from build123d import *

# Parameters (mm, degrees)
BOSS_EXTRUDE1_DEPTH = 1.5875
CUT_EXTRUDE1_DEPTH  = 5.08


with BuildPart() as part:
    # Sketch2 → Boss-Extrude1 (new body, symmetric)
    with BuildSketch(Plane.XY):
        Polygon((-31.75, -76.2), (-95.25, -76.2), (-31.75, 76.2), (31.75, 76.2), (31.75, -76.2), align=None)
    extrude(amount=BOSS_EXTRUDE1_DEPTH, both=True)

    # Sketch3 → Cut-Extrude1 (cut)
    with BuildSketch(Plane.XY.offset(1.5875)):
        with BuildLine():
            Line((-60.897552188, -22.755874748), (-42.901529882, -65.946328282))
            ThreePointArc((-42.901529882, -65.946328282), (-43.158162937, -68.594558042), (-45.503977694, -69.85))
            Line((-45.503977694, -69.85), (-81.496022306, -69.85))
            ThreePointArc((-81.496022306, -69.85), (-83.841837063, -68.594558042), (-84.098470118, -65.946328282))
            Line((-84.098470118, -65.946328282), (-66.102447812, -22.755874748))
            ThreePointArc((-66.102447812, -22.755874748), (-63.5, -21.020909541), (-60.897552188, -22.755874748))
        make_face()
        with BuildLine():
            ThreePointArc((-25.4, 30.353407686), (-23.133595378, 33.117976889), (-19.978233725, 31.437760941))
            Line((-19.978233725, 31.437760941), (-7.330980523, 1.084353255))
            ThreePointArc((-7.330980523, 1.084353255), (-7.114109872, 0), (-7.330980523, -1.084353255))
            Line((-7.330980523, -1.084353255), (-19.978233725, -31.437760941))
            ThreePointArc((-19.978233725, -31.437760941), (-23.133595378, -33.117976889), (-25.4, -30.353407686))
            Line((-25.4, -30.353407686), (-25.4, 30.353407686))
        make_face()
        with BuildLine():
            ThreePointArc((-20.598470118, 65.946328282), (-20.341837063, 68.594558042), (-17.996022306, 69.85))
            Line((-17.996022306, 69.85), (17.996022306, 69.85))
            ThreePointArc((17.996022306, 69.85), (20.341837063, 68.594558042), (20.598470118, 65.946328282))
            Line((20.598470118, 65.946328282), (2.602447812, 22.755874748))
            ThreePointArc((2.602447812, 22.755874748), (0, 21.020909541), (-2.602447812, 22.755874748))
            Line((-2.602447812, 22.755874748), (-20.598470118, 65.946328282))
        make_face()
        with BuildLine():
            ThreePointArc((-2.602447812, -22.755874748), (0, -21.020909541), (2.602447812, -22.755874748))
            Line((2.602447812, -22.755874748), (20.598470118, -65.946328282))
            ThreePointArc((20.598470118, -65.946328282), (20.341837063, -68.594558042), (17.996022306, -69.85))
            Line((17.996022306, -69.85), (-17.996022306, -69.85))
            ThreePointArc((-17.996022306, -69.85), (-20.341837063, -68.594558042), (-20.598470118, -65.946328282))
            Line((-20.598470118, -65.946328282), (-2.602447812, -22.755874748))
        make_face()
        with BuildLine():
            Line((-38.1, 30.353407686), (-38.1, -30.353407686))
            ThreePointArc((-38.1, -30.353407686), (-40.366404622, -33.117976889), (-43.521766275, -31.437760941))
            Line((-43.521766275, -31.437760941), (-56.169019477, -1.084353255))
            ThreePointArc((-56.169019477, -1.084353255), (-56.385890128, 0), (-56.169019477, 1.084353255))
            Line((-56.169019477, 1.084353255), (-43.521766275, 31.437760941))
            ThreePointArc((-43.521766275, 31.437760941), (-40.366404622, 33.117976889), (-38.1, 30.353407686))
        make_face()
        with BuildLine():
            Line((25.4, -30.353407686), (25.4, 30.353407686))
            ThreePointArc((25.4, 30.353407686), (23.133595378, 33.117976889), (19.978233725, 31.437760941))
            Line((19.978233725, 31.437760941), (7.330980523, 1.084353255))
            ThreePointArc((7.330980523, 1.084353255), (7.114109872, 0), (7.330980523, -1.084353255))
            Line((7.330980523, -1.084353255), (19.978233725, -31.437760941))
            ThreePointArc((19.978233725, -31.437760941), (23.133595378, -33.117976889), (25.4, -30.353407686))
        make_face()
    extrude(amount=-CUT_EXTRUDE1_DEPTH, mode=Mode.SUBTRACT)


solid = part.part
Design review of the part built by this model. Coordinates are the model's own, in mm. Coordinates: 2 decimals unless noted, no trailing zeros. Order: outer loops, then holes, each group sorted by start corner. A loop starts at its lowest first (then second) coordinate and runs counter-clockwise, first axis right, second up.
Item 1: Take a section at B-B, the plane x = 0.5. Write out the cut boundary in (y, z).
Item 2: Take a section at A-A, the plane y = -46. Write out the cut boundary in (x, z).
Item 3: Take a section at C-C, the plane z = -0.25. Count the separate pieces of the cut face and the enclosed holes in it, then the cut area to 3 significant figures.
Item 4: For pin 1 Ø1.6 at (x, z) = (-63.5, -0.5) entering from +Y; pin 2 Ø1.6 at (y, z) = (-14, 0.5) entering from -X, all flat-tipped, find the tip position at first contact; note any pin that passes through.
Item 5: The part is to be moulded in two halves that separate along X. For faces 1 (the flat face through (-52.026, -44.049, 0.022)), 2 (the flat face through (-63.944, -1.067, 0.022)), say which applies: pulls with the +X half, pulls with the -X half, needs draft (parallel to the pull), parting line crosses it, or undercut.
Item 6: For line 1 (X direction, y = -7.5, z = -1.15) (3 decimals); line 2 (X direction, y = 4, z = 1.1); line 3 (X direction, y = -67, z = 1), list the stretches that pass through material, from the lowest coordinate up.
Item 7: Take a section at D-D, the plane y = -28. Write out the cut boundary in (x, z).
The answers:
1. outline: (-76.2, -1.59) - (-69.85, -1.59) - (-69.85, 1.59) - (-76.2, 1.59) - close; (-21.07, -1.59) - (21.07, -1.59) - (21.07, 1.59) - (-21.07, 1.59) - close; (69.85, -1.59) - (76.2, -1.59) - (76.2, 1.59) - (69.85, 1.59) - close
2. outline: (-82.67, -1.59) - (-75.79, -1.59) - (-75.79, 1.59) - (-82.67, 1.59) - close; (-51.21, -1.59) - (-12.29, -1.59) - (-12.29, 1.59) - (-51.21, 1.59) - close; (12.29, -1.59) - (31.75, -1.59) - (31.75, 1.59) - (12.29, 1.59) - close
3. separate pieces: 1
3. enclosed holes: 6
3. area: 8,720 mm2
4. pin 1: stops at y = 1.92
4. pin 2: stops at x = -69.67
5. face 1: undercut
5. face 2: pulls with the -X half
6. line 1: x = -66.625 to -53.496, -38.1 to -25.4, -10.004 to 10.004, 25.4 to 31.75
6. line 2: x = -61.83 to -54.95, -38.1 to -25.4, -8.55 to 8.55, 25.4 to 31.75
6. line 3: x = -91.42 to -84.32, -42.68 to -20.82, 20.82 to 31.75
7. outline: (-75.17, -1.59) - (-68.29, -1.59) - (-68.29, 1.59) - (-75.17, 1.59) - close; (-58.71, -1.59) - (-44.95, -1.59) - (-44.95, 1.59) - (-58.71, 1.59) - close; (-38.1, -1.59) - (-25.4, -1.59) - (-25.4, 1.59) - (-38.1, 1.59) - close; (-18.55, -1.59) - (-4.79, -1.59) - (-4.79, 1.59) - (-18.55, 1.59) - close; (4.79, -1.59) - (18.55, -1.59) - (18.55, 1.59) - (4.79, 1.59) - close; (25.4, -1.59) - (31.75, -1.59) - (31.75, 1.59) - (25.4, 1.59) - close
